from build123d import *

# Parameters (mm, degrees)
SKETCH1_R           = 5
BOSS_EXTRUDE1_DEPTH = 22.63
SKETCH2_R           = 3.25
CUT_EXTRUDE1_DEPTH  = 9.652
SKETCH3_R           = 2.5
CUT_EXTRUDE2_DEPTH  = 9.978
SKETCH4_R           = 1.5
CUT_EXTRUDE3_DEPTH  = 3
BOSS_EXTRUDE3_START = -2
SKETCH5_R           = 5
BOSS_EXTRUDE3_DEPTH = 2


with BuildPart() as part:
    # Sketch1 → Boss-Extrude1 (new body)
    with BuildSketch(Plane(origin=(0, 0, 0), x_dir=(1, 0, 0), z_dir=(0, 1, 0))):
        with Locations(Location((0, 0, 0), (0, 0, 270))):
            Circle(SKETCH1_R)
    extrude(amount=BOSS_EXTRUDE1_DEPTH)

    # Sketch2 → Cut-Extrude1 (cut)
    with BuildSketch(Plane(origin=(0, 22.63, 0), x_dir=(1, 0, 0), z_dir=(0, 1, 0))):
        with Locations(Location((0, 0, 0), (0, 0, 270))):
            Circle(SKETCH2_R)
    extrude(amount=-CUT_EXTRUDE1_DEPTH, mode=Mode.SUBTRACT)

    # Sketch3 → Cut-Extrude2 (cut)
    with BuildSketch(Plane(origin=(0, 12.978, 0), x_dir=(1, 0, 0), z_dir=(0, 1, 0))):
        with Locations(Location((0, 0, 0), (0, 0, 270))):
            Circle(SKETCH3_R)
    extrude(amount=-CUT_EXTRUDE2_DEPTH, mode=Mode.SUBTRACT)

    # Sketch4 → Cut-Extrude3 (cut)
    with BuildSketch(Plane(origin=(0, 3, 0), x_dir=(1, 0, 0), z_dir=(0, 1, 0))):
        with Locations(Location((0, 0, 0), (0, 0, 270))):
            Circle(SKETCH4_R)
    extrude(amount=-CUT_EXTRUDE3_DEPTH, mode=Mode.SUBTRACT)

    # Sketch5 → Boss-Extrude3 (add)
    with BuildSketch(Plane(origin=(0, 22.63, 0), x_dir=(1, 0, 0), z_dir=(0, 1, 0)).offset(BOSS_EXTRUDE3_START)):
        with BuildLine():
            Line((6.25, -4.145780988), (6.25, 4.145780988))
            ThreePointArc((6.25, 4.145780988), (0, 7.5), (-6.25, 4.145780988))
            Line((-6.25, 4.145780988), (-6.25, -4.145780988))
            ThreePointArc((-6.25, -4.145780988), (0, -7.5), (6.25, -4.145780988))
        make_face()
        with Locations(Location((0, 0, 0), (0, 0, 270))):
            Circle(SKETCH5_R, mode=Mode.SUBTRACT)
    extrude(amount=BOSS_EXTRUDE3_DEPTH)


solid = part.part
Read the model definition and answer for the solid it produces. Units are mm, in the model's axes. A direction names the side the tool comes from. Give positions to 0.01 mm unless a question says otherwise; leave off trailing zeros. Write each loop counter-clockwise with the first axis right and the second up, starting at its lowest first coordinate (ties: lowest second). Pieces come first, ordered by that corner, then holes. Notation, with made-up numbers: (-10.75, 30) - (-5.75, 30) arc R18 ccw to (-5.75, 53) - close; hole circle Ø11 at (23.5, 37.5). An arc over 180 degrees is marked (long way). Use CSV: the item, a comma, the result in double quotes. Start each with the question number.
(1) Find section C-C (y = 8.5). Give the vertices of the cut face in (x, z), plus the area to 3 significant figures.
(2) Find section B-B (z = 0). Give the vertices of the cut face in (x, y), plus the area to 3 significant figures.
(3) For faces 1 (the flat face through (1.3, 20.63, -5.1)), 2 (the cylindrical face through (0.1, 21.6, -7.5)), 3 (the cylindrical face through (-2.44, 8.06, -0.54)), determine the directions among +Z, -Z, +X, -X, +Y, -Y from which every point of the face is accessible in a straight line to the end or side of a thin tool.
(4) Determine the mould class of faces 4 (the flat face through (1.2, 0, -1.2)), 5 (the cylindrical face through (-4.88, 10.17, -1.08)), 6 (the flat face through (-2, 12.978, 2)) for opening direction Z: +Z half, -Z half, draft (parallel to the pull), parting line (faces both ways), or undercut.
(5) Given P1, Ø6, axis at y = 4, z = -1, coming from the +X side; P2, Ø1, axis at y = 14, z = -4, coming from the +X side; P3, Ø3.5, axis at x = 0, z = 0, coming from the +Y side, each flat-ended and moving along its own axis, determine where each tip first touches the part or whether it passes through.
(6) Consider line 1 along X through (y, z) = (15, 0); line 2 along X through (y, z) = (1.3, 0); line 3 along Y through (x, z) = (-3.75, -5.75). Determine where each line is inside the solid, lowest interval first.
(7) Find section A-A (x = 0). Give the vertices of the cut face in (y, z), plus the area to 3 significant figures.
(8) Find section D-D (x = -2.25). Give the vertices of the cut face in (y, z).
Findings below:
1,outline,"circle Ø10 at (0, 0); hole circle Ø5 at (0, 0)"
1,area,"58.9 mm2"
2,outline,"(-6.25, 20.63) - (-5, 20.63) - (-5, 0) - (-1.5, 0) - (-1.5, 3) - (-2.5, 3) - (-2.5, 12.98) - (-3.25, 12.98) - (-3.25, 22.63) - (-6.25, 22.63) - close; (1.5, 0) - (5, 0) - (5, 20.63) - (6.25, 20.63) - (6.25, 22.63) - (3.25, 22.63) - (3.25, 12.98) - (2.5, 12.98) - (2.5, 3) - (1.5, 3) - close"
2,area,"110 mm2"
3,face 1,"-Y"
3,face 2,"-Z, +Y, -Y"
3,face 3,"+Y"
4,face 4,"draft"
4,face 5,"parting line"
4,face 6,"undercut"
5,P1,"x = 5"
5,P2,"x = 3.57"
5,P3,"y = 3"
6,line 1,"-5 to -3.25, 3.25 to 5"
6,line 2,"-5 to -1.5, 1.5 to 5"
6,line 3,"20.63 to 22.63"
7,outline,"(0, -5) - (20.63, -5) - (20.63, -7.5) - (22.63, -7.5) - (22.63, -3.25) - (12.98, -3.25) - (12.98, -2.5) - (3, -2.5) - (3, -1.5) - (0, -1.5) - close; (0, 1.5) - (3, 1.5) - (3, 2.5) - (12.98, 2.5) - (12.98, 3.25) - (22.63, 3.25) - (22.63, 7.5) - (20.63, 7.5) - (20.63, 5) - (0, 5) - close"
7,area,"115 mm2"
8,outline,"(0, -4.47) - (20.63, -4.47) - (20.63, -7.15) - (22.63, -7.15) - (22.63, -2.35) - (12.98, -2.35) - (12.98, -1.09) - (3, -1.09) - (3, 1.09) - (12.98, 1.09) - (12.98, 2.35) - (22.63, 2.35) - (22.63, 7.15) - (20.63, 7.15) - (20.63, 4.47) - (0, 4.47) - close"
